Geometry check sheet. Reference: the model listing, model coordinates, mm. A direction names the side the tool comes from. Give positions to 0.01 mm unless a question says otherwise; leave off trailing zeros. Write each loop counter-clockwise with the first axis right and the second up, starting at its lowest first coordinate (ties: lowest second). Pieces come first, ordered by that corner, then holes. Notation, with made-up numbers: (36.25, 38.25) - (40.25, 38.25) arc R27 ccw to (40.25, 55.25) - close; hole circle Ø1 at (64.25, 62). An arc over 180 degrees is marked (long way). One line per question, with ' | ' between items. Start each with the question number.
Q1. Section check B-B on x = 6.75. Record the boundary of the cut face in (y, z) (3 decimals).
Q2. Section check D-D on x = 2.5. Record the boundary of the cut face in (y, z) (3 decimals), and give its area (3 significant figures).
Q3. Thickness scan on L1, parallel to X at y = -3, z = -3.5; L2, parallel to Y at x = -2, z = -3.5; L3, parallel to Y at x = 4.5, z = -3.25. Record the ranges inside material, lowest first. Write a range as [from, to].
Q4. Section check A-A on y = 0. Record the boundary of the cut face in (x, z).
Q5. Gauge pin test, flat ends, axial feed: P1, Ø1.7, axis at x = 3.5, z = -5.5, coming from the -Y side; P2, Ø3.5, axis at x = -4, z = -5.5, coming from the -Y side; P3, Ø6, axis at x = -5, y = -7.5, coming from the +Z side. Record the tip position at first contact, or that the pin passes through.
Q6. Release check for a two-part mould opening along Y. For faces 4 (the face through (-11.65, -2.9, -9.57)), 5 (the face through (13, 1.87, -2.13)), 6 (the face through (-10.685, -1, 6)), 7 (the face through (0, -0.41, -5)) record: +Y half, -Y half, draft (parallel to the pull), parting line (faces both ways), or undercut.
Q7. Set-up check for faces 1 (the face through (12, 0.4, 6)), 2 (the face through (-10.685, -4, -1)), 3 (the face through (0, 2, -3.075)): record each of +Z, -Z, +X, -X, +Y, -Y from which the full face is reachable in a straight line by a thin tool's end or side.
```python
from build123d import *

# Parameters (mm, degrees)
CUT_EXTRUDE1_DEPTH            = 4.5
CUT_EXTRUDE4_REACH            = 31.597
CUT_EXTRUDE5_START            = -2.314830862
CUT_EXTRUDE5_DEPTH            = 2.314830862
CUT_EXTRUDE6_REACH            = 22.975
CUT_EXTRUDE6_END_MAJOR_RADIUS = 23
CUT_EXTRUDE6_END_MINOR_RADIUS = 17
SKETCH10_W                    = 21.370338276
SKETCH10_H                    = 4.1


with BuildPart() as part:
    # Sketch1 → Revolve1 (revolve)
    with BuildSketch(Plane(origin=(0, 0, 0), x_dir=(1, 0, 0), z_dir=(0, 1, 0)), mode=Mode.PRIVATE) as revolve1_sk:
        with BuildLine():
            Line((11.313708499, 10), (12, 10))
            ThreePointArc((12, 10), (12.707106781, 9.707106781), (13, 9))
            Line((13, 9), (13, 0))
            Line((13, 0), (-13, 0))
            Line((-13, 0), (-13, 9))
            ThreePointArc((-13, 9), (-12.707106781, 9.707106781), (-12, 10))
            Line((-12, 10), (-11.313708499, 10))
            ThreePointArc((-11.313708499, 10), (-10.980375166, 9.942809042), (-10.685169138, 9.777777778))
            ThreePointArc((-10.685169138, 9.777777778), (0, 6), (10.685169138, 9.777777778))
            ThreePointArc((10.685169138, 9.777777778), (10.980375166, 9.942809042), (11.313708499, 10))
        make_face()
    revolve(revolve1_sk.sketch.rotate(Axis((-13, 0, 0), (1, 0, 0)), 180), axis=Axis((-13, 0, 0), (1, 0, 0)))

    # Sketch3 → Cut-Extrude1 (cut, symmetric)
    with BuildSketch(Plane(origin=(0, 0, 0), x_dir=(1, 0, 0), z_dir=(0, 1, 0))):
        with BuildLine():
            Line((-9.147669138, -10), (9.147669138, -10))
            Line((9.147669138, -10), (10.685169138, -10))
            Line((10.685169138, -10), (10.685169138, 2))
            Line((10.685169138, 2), (9.969897363, 2))
            ThreePointArc((9.969897363, 2), (9.287033253, 1.817172167), (8.786871434, 1.31760479))
            ThreePointArc((8.786871434, 1.31760479), (0, -3.750854676), (-8.786871434, 1.31760479))
            ThreePointArc((-8.786871434, 1.31760479), (-9.287033253, 1.817172167), (-9.969897363, 2))
            Line((-9.969897363, 2), (-10.685169138, 2))
            Line((-10.685169138, 2), (-10.685169138, -10))
            Line((-10.685169138, -10), (-9.147669138, -10))
        make_face()
    extrude(amount=CUT_EXTRUDE1_DEPTH, both=True, mode=Mode.SUBTRACT)

    # Cut-Extrude4: up to this face of the body (flat: up to its plane)
    cut_extrude4_end = Plane(part.part.faces().sort_by_distance((-10.685169138, 0, 3.71495774))[0])
    # Sketch6 → Cut-Extrude4 (cut, up to the picked face)
    with BuildSketch(Plane.ZY.offset(13), mode=Mode.PRIVATE) as cut_extrude4_sk1:
        with BuildLine():
            Line((1.075, -4.5), (2.6125, -4.5))
            ThreePointArc((2.6125, -4.5), (4.6625, -2.45), (2.6125, -0.4))
            Line((2.6125, -0.4), (1.5875, -0.4))
            ThreePointArc((1.5875, -0.4), (1.1875, 0), (1.5875, 0.4))
            Line((1.5875, 0.4), (9.991996797, 0.4))
            ThreePointArc((9.991996797, 0.4), (9.680686562, 2.506852148), (8.93028555, 4.5))
            Line((8.93028555, 4.5), (1.075, 4.5))
            ThreePointArc((1.075, 4.5), (-1.099353352, 3.599353352), (-2, 1.425))
            Line((-2, 1.425), (-2, -1.425))
            ThreePointArc((-2, -1.425), (-1.099353352, -3.599353352), (1.075, -4.5))
        make_face()
    cut_extrude4_tool1 = split(extrude(cut_extrude4_sk1.sketch, amount=-CUT_EXTRUDE4_REACH, mode=Mode.PRIVATE), bisect_by=cut_extrude4_end, keep=Keep.BOTH, mode=Mode.PRIVATE)
    add(cut_extrude4_tool1.solids().sort_by(Axis((-13, 0.735249, 2.995386), (1, 0, 0)))[0], mode=Mode.SUBTRACT)

    # Sketch8 → Cut-Extrude5 (cut)
    with BuildSketch(Plane(origin=(13, 0, 0), x_dir=(0, 0, -1), z_dir=(1, 0, 0)).offset(CUT_EXTRUDE5_START)):
        with BuildLine():
            Line((-1.5875, 0.4), (-9.991996797, 0.4))
            ThreePointArc((-9.991996797, 0.4), (-9.680686562, 2.506852148), (-8.93028555, 4.5))
            Line((-8.93028555, 4.5), (-1.075, 4.5))
            ThreePointArc((-1.075, 4.5), (1.099353352, 3.599353352), (2, 1.425))
            Line((2, 1.425), (2, -1.425))
            ThreePointArc((2, -1.425), (1.099353352, -3.599353352), (-1.075, -4.5))
            Line((-1.075, -4.5), (-2.6125, -4.5))
            ThreePointArc((-2.6125, -4.5), (-4.6625, -2.45), (-2.6125, -0.4))
            Line((-2.6125, -0.4), (-1.5875, -0.4))
            ThreePointArc((-1.5875, -0.4), (-1.1875, 0), (-1.5875, 0.4))
        make_face()
    extrude(amount=CUT_EXTRUDE5_DEPTH, mode=Mode.SUBTRACT)

    # Cut-Extrude6: up to this torus (the profile starts outside it)
    cut_extrude6_end = Plane(origin=(0, 0, 0), z_dir=(-1, 0, 0)) * Torus(CUT_EXTRUDE6_END_MAJOR_RADIUS, CUT_EXTRUDE6_END_MINOR_RADIUS, mode=Mode.PRIVATE)
    # Sketch10 → Cut-Extrude6 (cut, up to the surface)
    with BuildSketch(Plane.XY.offset(-3.075), mode=Mode.PRIVATE) as cut_extrude6_sk1:
        with Locations((0, 2.46)):
            Rectangle(SKETCH10_W, SKETCH10_H)
    cut_extrude6_tool1 = extrude(cut_extrude6_sk1.sketch, amount=-CUT_EXTRUDE6_REACH, mode=Mode.PRIVATE) - cut_extrude6_end
    add(cut_extrude6_tool1.solids().sort_by_distance((0, 2.46, -3.075))[0], mode=Mode.SUBTRACT)
    # Sketch10 → Cut-Extrude6 (cut, up to the surface)
    with BuildSketch(Plane.XY.offset(-3.075), mode=Mode.PRIVATE) as cut_extrude6_sk2:
        with Locations((0, -2.46)):
            Rectangle(SKETCH10_W, SKETCH10_H)
    cut_extrude6_tool2 = extrude(cut_extrude6_sk2.sketch, amount=-CUT_EXTRUDE6_REACH, mode=Mode.PRIVATE) - cut_extrude6_end
    add(cut_extrude6_tool2.solids().sort_by_distance((0, -2.46, -3.075))[0], mode=Mode.SUBTRACT)


solid = part.part
```
Working result:
1) outline: (-4.51, -5.864) - (-4.51, -3.075) - (-0.41, -3.075) - (-0.41, -7.386) arc R7.398 ccw to (0.41, -7.386) - (0.41, -3.075) - (4.51, -3.075) - (4.51, -5.864) arc R7.398 ccw to (4.5, 5.871) - (4.5, 1.181) - (-4.5, 1.181) - (-4.5, 5.871) arc R7.398 ccw to start
2) outline: (-4.51, -4.232) - (-4.51, -3.075) - (-0.41, -3.075) - (-0.41, -6.171) arc R6.185 ccw to (0.41, -6.171) - (0.41, -3.075) - (4.51, -3.075) - (4.51, -4.232) arc R6.185 ccw to (4.5, 4.243) - (4.5, 3.438) - (-4.5, 3.438) - (-4.5, 4.243) arc R6.185 ccw to start | area: 80.8 mm2
3) L1: x = [-13, -10.69], [10.69, 13] | L2: y = [-5.02, -4.51], [-0.41, 0.41], [4.51, 5.02] | L3: y = [-5.75, -4.51], [-0.41, 0.41], [4.51, 5.75]
4) outline: (-13, -9) arc R1 ccw to (-12, -10) - (-11.31, -10) arc R1 ccw to (-10.69, -9.78) arc R17 cw to (10.69, -9.78) arc R1 ccw to (11.31, -10) - (12, -10) arc R1 ccw to (13, -9) - (13, -2) - (9.97, -2) arc R1.37 cw to (8.79, -1.32) arc R10.15 ccw to (-8.79, -1.32) arc R1.37 cw to (-9.97, -2) - (-13, -2) - close; (-13, 1.19) - (-10.69, 1.19) - (-10.69, 9.78) arc R1 ccw to (-11.31, 10) - (-12, 10) arc R1 ccw to (-13, 9) - close; (10.69, 1.19) - (13, 1.19) - (13, 9) arc R1 ccw to (12, 10) - (11.31, 10) arc R1 ccw to (10.69, 9.78) - close
5) P1: stops at y = -0.41 | P2: stops at y = -5.41 | P3: stops at z = 5.4
6) face 4: parting line | face 5: draft | face 6: undercut | face 7: undercut
7) face 1: +Z, +X | face 2: +Z | face 3: -Z
